Design review of the part built by this model. Coordinates are the model's own, in mm. A direction names the side the tool comes from. Give positions to 0.01 mm unless a question says otherwise; leave off trailing zeros. Order: outer loops, then holes, each group sorted by start corner. A loop starts at its lowest first (then second) coordinate and runs counter-clockwise, first axis right, second up. Notation, with made-up numbers: (-25, 66.25) -> (-17, 66.25) arc R19 cw to (-17, 86.25) -> close; hole circle Ø1 at (6, 1.25). An arc over 180 degrees is marked (long way). One line per item, written item: value.
from build123d import *

# Parameters (mm, degrees)
SKETCH_1_R          = 2
SKETCH_1_R_2        = 11
EXTRUDE_1_DEPTH     = 4
CUT_EXTRUDE_2_DEPTH = 4


with BuildPart() as part:
    # 草图1 → 凸台-拉伸1 (new body)
    with BuildSketch(Plane.XY):
        Polygon((149, 64.5), (145, 64.5), (145, 37), (141, 37), (141, 29), (145, 29), (145, 6.9), (151.5, 6.9), (180.5, 6.9), (180.5, 2.9), (188.5, 2.9), (188.5, 6.9), (216, 6.9), (216, 10.9), (214.65, 10.9), (214.65, 13.5), (216, 13.5), (216, 15.5), (219, 15.5), (219, 13.5), (220.35, 13.5), (220.35, 10.9), (219, 10.9), (219, 6.9), (246.5, 6.9), (246.5, 2.9), (254.5, 2.9), (254.5, 6.9), (283.5, 6.9), (290, 6.9), (290, 29), (294, 29), (294, 37), (290, 37), (290, 64.5), (286, 64.5), (286, 63.15), (283.4, 63.15), (283.4, 64.5), (281.4, 64.5), (281.4, 67.5), (283.4, 67.5), (283.4, 68.85), (286, 68.85), (286, 67.5), (290, 67.5), (290, 95), (294, 95), (294, 103), (290, 103), (290, 132), (145, 132), (145, 103), (141, 103), (141, 95), (145, 95), (145, 67.5), (149, 67.5), (149, 68.85), (151.6, 68.85), (151.6, 67.5), (153.6, 67.5), (153.6, 64.5), (151.6, 64.5), (151.6, 63.15), (149, 63.15), align=None)
        with Locations((197.5, 26)):
            Circle(SKETCH_1_R, mode=Mode.SUBTRACT)
        with Locations((202.014361492, 50.514361492)):
            Circle(SKETCH_1_R, mode=Mode.SUBTRACT)
        with Locations((195.6, 66)):
            Circle(SKETCH_1_R, mode=Mode.SUBTRACT)
        with Locations((237.5, 26)):
            Circle(SKETCH_1_R, mode=Mode.SUBTRACT)
        with Locations((217.5, 44.1)):
            Circle(SKETCH_1_R, mode=Mode.SUBTRACT)
        with Locations((232.985638508, 50.514361492)):
            Circle(SKETCH_1_R, mode=Mode.SUBTRACT)
        with Locations((217.5, 66)):
            Circle(SKETCH_1_R_2, mode=Mode.SUBTRACT)
        with Locations((239.4, 66)):
            Circle(SKETCH_1_R, mode=Mode.SUBTRACT)
        with Locations((202.014361492, 81.485638508)):
            Circle(SKETCH_1_R, mode=Mode.SUBTRACT)
        with Locations((197.5, 106)):
            Circle(SKETCH_1_R, mode=Mode.SUBTRACT)
        with Locations((232.985638508, 81.485638508)):
            Circle(SKETCH_1_R, mode=Mode.SUBTRACT)
        with Locations((217.5, 87.9)):
            Circle(SKETCH_1_R, mode=Mode.SUBTRACT)
        with Locations((237.5, 106)):
            Circle(SKETCH_1_R, mode=Mode.SUBTRACT)
    extrude(amount=EXTRUDE_1_DEPTH)

    # 草图3 → 切除-拉伸2 (cut)
    with BuildSketch(Plane(origin=(0, 0, 0), x_dir=(-1, 0, 0), z_dir=(0, 0, -1))):
        with BuildLine():
            Line((-255.447331922, 61), (-272.4, 61))
            ThreePointArc((-272.4, 61), (-275.228427125, 59.828427125), (-276.4, 57))
            Line((-276.4, 57), (-276.4, 32.858450899))
            ThreePointArc((-276.4, 32.858450899), (-274.116182938, 29.24531983), (-269.872641938, 29.758053953))
            Line((-269.872641938, 29.758053953), (-250.07214558, 45.898872363))
            ThreePointArc((-250.07214558, 45.898872363), (-248.6940963, 48.134518776), (-248.999554551, 50.742933995))
            ThreePointArc((-248.999554551, 50.742933995), (-250.473448142, 54.263232234), (-251.555297879, 57.923076923))
            ThreePointArc((-251.555297879, 57.923076923), (-252.96663723, 60.137858162), (-255.447331922, 61))
        make_face()
        with BuildLine():
            Line((-269.707278747, 106.765103218), (-248.927132883, 87.848004914))
            ThreePointArc((-248.927132883, 87.848004914), (-247.673089718, 85.54051484), (-248.120381917, 82.952646144))
            ThreePointArc((-248.120381917, 82.952646144), (-250.140932956, 78.632082004), (-251.555297879, 74.076923077))
            ThreePointArc((-251.555297879, 74.076923077), (-252.96663723, 71.862141838), (-255.447331922, 71))
            Line((-255.447331922, 71), (-272.4, 71))
            ThreePointArc((-272.4, 71), (-275.228427125, 72.171572875), (-276.4, 75))
            Line((-276.4, 75), (-276.4, 103.807189721))
            ThreePointArc((-276.4, 103.807189721), (-274.016959336, 107.465801822), (-269.707278747, 106.765103218))
        make_face()
        with BuildLine():
            Line((-158.6, 57), (-158.6, 32.858450899))
            ThreePointArc((-158.6, 32.858450899), (-160.883817062, 29.24531983), (-165.127358062, 29.758053953))
            Line((-165.127358062, 29.758053953), (-184.92785442, 45.898872363))
            ThreePointArc((-184.92785442, 45.898872363), (-186.3059037, 48.134518776), (-186.000445449, 50.742933995))
            ThreePointArc((-186.000445449, 50.742933995), (-184.526551858, 54.263232234), (-183.444702121, 57.923076923))
            ThreePointArc((-183.444702121, 57.923076923), (-182.03336277, 60.137858162), (-179.552668078, 61))
            Line((-179.552668078, 61), (-162.6, 61))
            ThreePointArc((-162.6, 61), (-159.771572875, 59.828427125), (-158.6, 57))
        make_face()
        with BuildLine():
            Line((-179.552668078, 71), (-162.6, 71))
            ThreePointArc((-162.6, 71), (-159.771572875, 72.171572875), (-158.6, 75))
            Line((-158.6, 75), (-158.6, 103.807189721))
            ThreePointArc((-158.6, 103.807189721), (-160.983040664, 107.465801822), (-165.292721253, 106.765103218))
            Line((-165.292721253, 106.765103218), (-186.072867117, 87.848004914))
            ThreePointArc((-186.072867117, 87.848004914), (-187.326910282, 85.54051484), (-186.879618083, 82.952646144))
            ThreePointArc((-186.879618083, 82.952646144), (-184.859067044, 78.632082004), (-183.444702121, 74.076923077))
            ThreePointArc((-183.444702121, 74.076923077), (-182.03336277, 71.862141838), (-179.552668078, 71))
        make_face()
        with BuildLine():
            Line((-261.576319533, 125), (-173.423680467, 125))
            ThreePointArc((-173.423680467, 125), (-169.693288129, 122.443666515), (-170.730959214, 118.042086503))
            Line((-170.730959214, 118.042086503), (-179.92985273, 109.667921372))
            ThreePointArc((-179.92985273, 109.667921372), (-181.961826365, 108.680785745), (-184.204551796, 108.951961409))
            ThreePointArc((-184.204551796, 108.951961409), (-217.5, 115.815856239), (-250.795448204, 108.951961409))
            ThreePointArc((-250.795448204, 108.951961409), (-253.038173635, 108.680785745), (-255.07014727, 109.667921372))
            Line((-255.07014727, 109.667921372), (-264.269040786, 118.042086503))
            ThreePointArc((-264.269040786, 118.042086503), (-265.306711871, 122.443666515), (-261.576319533, 125))
        make_face()
    extrude(amount=-CUT_EXTRUDE_2_DEPTH, mode=Mode.SUBTRACT)


solid = part.part
Item 1: Add section B-B on y = 44.1. Give the boundary of the cut face in (x, z), plus the area to 3 significant figures.
Returned:
outline: (145, 0) -> (158.6, 0) -> (158.6, 4) -> (145, 4) -> close; (182.72, 0) -> (215.5, 0) -> (215.5, 4) -> (182.72, 4) -> close; (219.5, 0) -> (252.28, 0) -> (252.28, 4) -> (219.5, 4) -> close; (276.4, 0) -> (290, 0) -> (290, 4) -> (276.4, 4) -> close
area: 371 mm²
Item 2: Add section C-C on z = 2.9. Count the separate pieces of the cut face and the enclosed holes in it, plus the area to 3 significant figures.
Returned:
separate pieces: 1
enclosed holes: 18
area: 13,700 mm²
Item 3: Clearance check with flat-ended pins moving along their axes: P1, Ø1.1, axis at y = 68.5, z = 2.5, coming from the +X side; P2, Ø3.5, axis at x = 239.4, y = 66, coming from the -Z side; P3, Ø2, axis at y = 14.5, z = 2.5, coming from the -X side. State where each tip first meets the part, or that it passes through.
Returned:
P1: x = 290
P2: through
P3: x = 145
Item 4: To check wall thickness, follow line 1 along Y through (x, z) = (217.5, 2.1); line 2 along X through (y, z) = (14.5, 1.1); line 3 along X through (y, z) = (97, 1.55). State the ranges of each line that lie inside material, in increasing order. Write a range as from..to.
Returned:
line 1: 15.5..42.1, 46.1..55, 77..85.9, 89.9..115.82, 125..132
line 2: 145..216, 219..290
line 3: 141..158.6, 176.02..258.98, 276.4..294
Item 5: Draft analysis for pull direction X (two halves, no side actions). For faces 1 (the flat face through (294, 99, 2)), 2 (the flat face through (141, 33, 2)), 3 (the flat face through (175.537, 97.439, 1.972)), state which applies: pulls with the +X half, pulls with the -X half, needs draft (parallel to the pull), parting line crosses it, or undercut.
Returned:
face 1: pulls with the +X half
face 2: pulls with the -X half
face 3: undercut
Item 6: Add section A-A on y = 26. Give the boundary of the cut face in (x, z), plus the area to 3 significant figures.
Returned:
outline: (145, 0) -> (195.5, 0) -> (195.5, 4) -> (145, 4) -> close; (199.5, 0) -> (235.5, 0) -> (235.5, 4) -> (199.5, 4) -> close; (239.5, 0) -> (290, 0) -> (290, 4) -> (239.5, 4) -> close
area: 548 mm²
Item 7: Machinability: for faces 4 (the flat face through (254.5, 5, 2)), 5 (the cylindrical face through (184.545, 54.213, 1.972)), 6 (the flat face through (292, 103, 2)), which of the approach directions +Z, -Z, +X, -X, +Y, -Y give a long, thin tool a straight path to every point of the face, cutting with its end or side? Answer none if there is none.
Returned:
face 4: +Z, -Z, +X, -Y
face 5: +Z, -Z
face 6: +Z, -Z, +X, +Y
